Could you check a few things on this drawing? It's one solid part, dimensions in mm from its lowest x, y, z. A direction names the side the tool comes from. Round coordinates to 2 decimals unless told otherwise and drop trailing zeros. Loops run counter-clockwise (first coordinate to the right, second up) from the corner with the lowest first, then second, coordinate; pieces in that order, holes last.
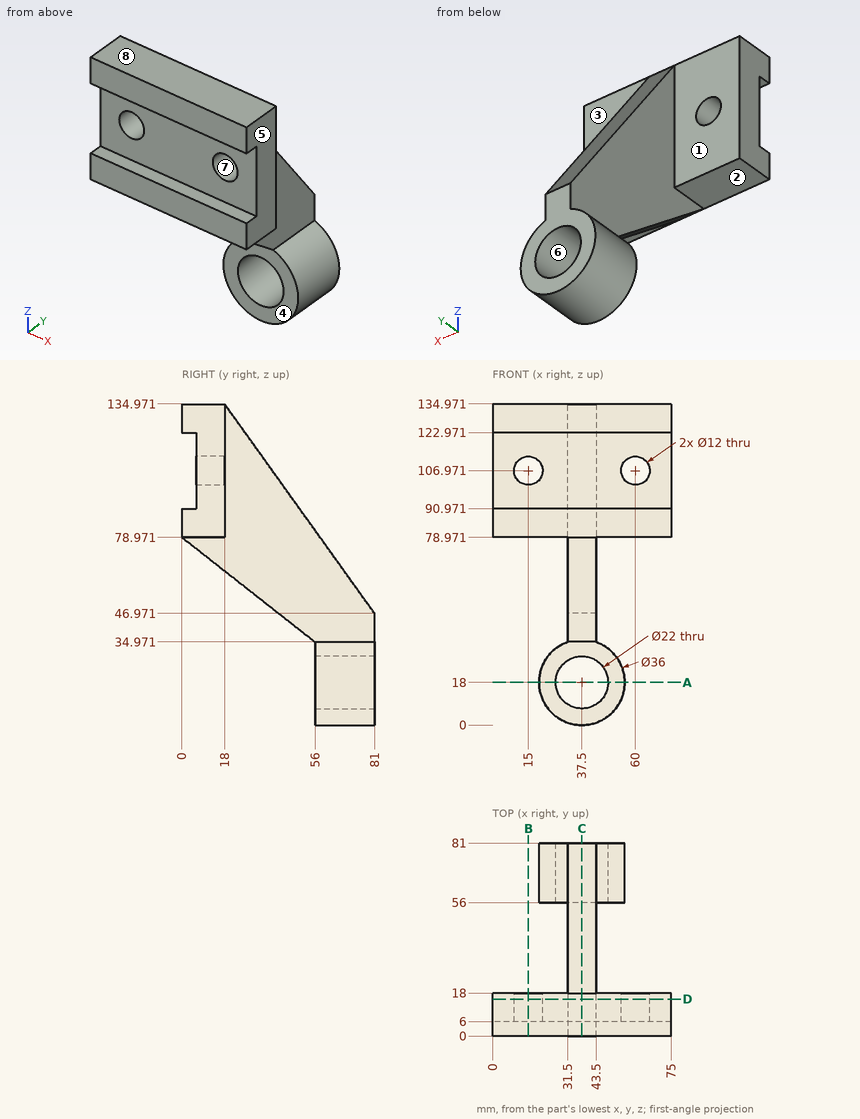
(1) Suppose I cut it at D-D (y = 15.5). Write out the boundary of the cut face in (x, z).
(2) If I drill on line 1 (X direction, y = 20.5, z = 66); line 2 (Y direction, x = 53, z = 119); line 3 (Y direction, x = 45, z = 90.5), over which ranges is the centre line in solid material (lowest first)?
(3) Suppose I cut it at A-A (z = 18). Write out the boundary of the cut face in (x, y), then the cut area to 3 significant figures.
(4) Suppose I cut it at B-B (x = 15). Write out the boundary of the cut face in (y, z).
(5) For pin 1 (5 mm diameter, centred on x = 34.5, y = 3.5, fed in from -Z) (1 decimal); pin 2 (25 mm diameter, centred on x = 15, z = 114.5, fed in from +Y); pin 3 (6 mm diameter, centred on x = 23.5, z = 121, fed in from -Y); pin 4 (14.5 mm diameter, centred on x = 60.5, y = 7.5, fed in from -Z), each with a flat end and sliding along its axis, tell me the tip position at first contact or that it passes through.
(6) Suppose I cut it at C-C (x = 37.5). Write out the boundary of the cut face in (y, z).
(7) Which directions (+Z, -Z, +X, -X, +Y, -Y) give clear straight access to the entire face, cutting with the end or side of a thin tool? Please do the marked faces 1, 2, 3 and 4.
(8) We'd pull the mould along Z, two halves only. Please class the marked faces 5, 6, 7 and 8: released by +Z, released by -Z, zero draft, split by the parting line, or undercut.
Check result:
1. outline: (0, 78.97) - (31.5, 78.97) - (31.5, 66.79) - (43.5, 66.79) - (43.5, 78.97) - (75, 78.97) - (75, 134.97) - (0, 134.97) - close; hole circle Ø12 at (15, 106.97); hole circle Ø12 at (60, 106.97)
2. line 1: x = 31.5 to 43.5
2. line 2: y = 6 to 18
2. line 3: y = 0 to 18
3. outline: (19.5, 56) - (26.5, 56) - (26.5, 81) - (19.5, 81) - close; (48.5, 56) - (55.5, 56) - (55.5, 81) - (48.5, 81) - close
3. area: 350 mm2
4. outline: (0, 78.97) - (18, 78.97) - (18, 100.97) - (6, 100.97) - (6, 90.97) - (0, 90.97) - close; (0, 122.97) - (6, 122.97) - (6, 112.97) - (18, 112.97) - (18, 134.97) - (0, 134.97) - close
5. pin 1: stops at z = 74.3
5. pin 2: stops at y = 18
5. pin 3: stops at y = 0
5. pin 4: stops at z = 78.97
6. outline: (0, 78.97) - (56, 34.97) - (56, 29) - (81, 29) - (81, 46.97) - (18, 134.97) - (0, 134.97) - (0, 122.97) - (6, 122.97) - (6, 90.97) - (0, 90.97) - close; (56, 0) - (81, 0) - (81, 7) - (56, 7) - close
7. face 1: +Z, -Z, -X, +Y
7. face 2: -Z, -X, +Y, -Y
7. face 3: +Z, -Z, +X, +Y
7. face 4: -Z, +X, -X, -Y
8. face 5: zero draft
8. face 6: undercut
8. face 7: undercut
8. face 8: released by +Z
